Work out the finished part from the listing and answer in its coordinate system (mm). A direction names the side the tool comes from. Give positions to 0.01 mm unless a question says otherwise; leave off trailing zeros. Loops run counter-clockwise (first coordinate to the right, second up) from the corner with the lowest first, then second, coordinate; pieces in that order, holes last. Notation, with made-up numbers: M 88,-19.5 L 105,-19.5 A28 ccw 105,-0.5 Z; hole C 14,-39 d1. An arc over 180 degrees is marked long. Answer as a JSON object with one key per item and string values. Group by question number.
```python
from build123d import *

# Parameters (mm, degrees)
BOSS_EXTRUDE1_DEPTH = 3
BOSS_EXTRUDE2_DEPTH = 41
BOSS_EXTRUDE3_DEPTH = 2
SKETCH5_R           = 4.5
CUT_EXTRUDE1_DEPTH  = 2


with BuildPart() as part:
    # Sketch1 → Boss-Extrude1 (new body)
    with BuildSketch(Plane(origin=(0, 0, 0), x_dir=(1, 0, 0), z_dir=(0, 1, 0))):
        with BuildLine():
            Line((1.5, 0), (28.5, 0))
            ThreePointArc((28.5, 0), (29.560660172, 0.439339828), (30, 1.5))
            Line((30, 1.5), (30, 18.5))
            ThreePointArc((30, 18.5), (29.560660172, 19.560660172), (28.5, 20))
            Line((28.5, 20), (1.5, 20))
            ThreePointArc((1.5, 20), (0.439339828, 19.560660172), (0, 18.5))
            Line((0, 18.5), (0, 1.5))
            ThreePointArc((0, 1.5), (0.439339828, 0.439339828), (1.5, 0))
        make_face()
    extrude(amount=BOSS_EXTRUDE1_DEPTH)

    # Sketch3 → Boss-Extrude2 (add)
    with BuildSketch(Plane(origin=(0, 3, 0), x_dir=(1, 0, 0), z_dir=(0, 1, 0))):
        with BuildLine():
            Line((10.5, 5), (19.5, 5))
            ThreePointArc((19.5, 5), (19.853553391, 5.146446609), (20, 5.5))
            Line((20, 5.5), (20, 14.5))
            ThreePointArc((20, 14.5), (19.853553391, 14.853553391), (19.5, 15))
            Line((19.5, 15), (10.5, 15))
            ThreePointArc((10.5, 15), (10.146446609, 14.853553391), (10, 14.5))
            Line((10, 14.5), (10, 5.5))
            ThreePointArc((10, 5.5), (10.146446609, 5.146446609), (10.5, 5))
        make_face()
    extrude(amount=BOSS_EXTRUDE2_DEPTH)

    # Sketch4 → Boss-Extrude3 (add)
    with BuildSketch(Plane(origin=(0, 44, 0), x_dir=(1, 0, 0), z_dir=(0, 1, 0))):
        with BuildLine():
            Line((33, -22.5), (-3, -22.5))
            ThreePointArc((-3, -22.5), (-4.414213562, -21.914213562), (-5, -20.5))
            Line((-5, -20.5), (-5, 40.5))
            ThreePointArc((-5, 40.5), (-4.414213562, 41.914213562), (-3, 42.5))
            Line((-3, 42.5), (33, 42.5))
            ThreePointArc((33, 42.5), (34.414213562, 41.914213562), (35, 40.5))
            Line((35, 40.5), (35, -20.5))
            ThreePointArc((35, -20.5), (34.414213562, -21.914213562), (33, -22.5))
        make_face()
    extrude(amount=BOSS_EXTRUDE3_DEPTH)

    # Sketch5 → Cut-Extrude1 (cut)
    with BuildSketch(Plane(origin=(0, 46, 0), x_dir=(1, 0, 0), z_dir=(0, 1, 0))):
        with Locations(Location((15, 27.5, 0), (0, 0, 270))):
            Circle(SKETCH5_R)
        with Locations(Location((15, -7.5, 0), (0, 0, 270))):
            Circle(SKETCH5_R)
    extrude(amount=-CUT_EXTRUDE1_DEPTH, mode=Mode.SUBTRACT)


solid = part.part
```
Item 1: A cutting plane is placed at C-C (x = 15). Determine the outline of the cut face in (y, z), and give its area (3 significant figures).
Item 2: For a pull along Y with two mould halves and no side action, classify faces 4 (the cylindrical face through (34.43, 44.99, 21.9)), 5 (the flat face through (15, 0, -10)), 6 (the flat face through (15, 23, -15)) as pulls with the +Y half, pulls with the -Y half, needs draft (parallel to the pull), parting line crosses it, or undercut.
Item 3: A cutting plane is placed at A-A (x = 22.5). Determine the outline of the cut face in (y, z).
Item 4: A cutting plane is placed at B-B (z = -27.5). Determine the outline of the cut face in (x, y).
Item 5: Given pin 1 Ø12 at (y, z) = (12.5, -21.5) entering from +X; pin 2 Ø1.5 at (y, z) = (1, -10) entering from +X; pin 3 Ø2.5 at (y, z) = (29, -9) entering from -X; pin 4 Ø10 at (x, y) = (18, 34) entering from +Z, each flat-ended and moving along its own axis, determine where each tip first touches the part or whether it passes through.
Item 6: A tool of negligible diameter and unlimited length cuts with its end or side. For faces 1 (the cylindrical face through (29.55, 1.48, -0.43)), 2 (the cylindrical face through (0.43, 1.48, -0.45)), 3 (the flat face through (0, 1, -10)), from which of +Z, -Z, +X, -X, +Y, -Y can it reach the whole face along a straight path? Write none if from no direction.
Item 7: A cutting plane is placed at D-D (y = 41). Determine the outline of the cut face in (x, z), and give its area (3 significant figures).
Item 8: Find the intervals of material crossed by probe 1 along X at (y, z) = (45.3, -27.5); probe 2 along Y at (x, z) = (1.5, -16); probe 3 along Y at (x, z) = (7, 0.5), in increasing order. Write a range as [from, to].
The answers:
{
 "1": {"outline": "M 0,-20 L 3,-20 L 3,-15 L 44,-15 L 44,-23 L 46,-23 L 46,3 L 44,3 L 44,-5 L 3,-5 L 3,0 L 0,0 Z; M 44,-42.5 L 46,-42.5 L 46,-32 L 44,-32 Z; M 44,12 L 46,12 L 46,22.5 L 44,22.5 Z", "area": "564 mm^2"},
 "2": {"face 4": "needs draft", "face 5": "pulls with the -Y half", "face 6": "undercut"},
 "3": {"outline": "M 0,-20 L 3,-20 L 3,0 L 0,0 Z; M 44,-42.5 L 46,-42.5 L 46,22.5 L 44,22.5 Z"},
 "4": {"outline": "M -5,44 L 10.5,44 L 10.5,46 L -5,46 Z; M 19.5,44 L 35,44 L 35,46 L 19.5,46 Z"},
 "5": {"pin 1": "passes through", "pin 2": "stops at x = 30", "pin 3": "stops at x = 10", "pin 4": "stops at z = -5"},
 "6": {"face 1": "+Z, +X, -Y", "face 2": "+Z, -X, -Y", "face 3": "+Z, -Z, -X, -Y"},
 "7": {"outline": "M 10,-14.5 A0.5 ccw 10.5,-15 L 19.5,-15 A0.5 ccw 20,-14.5 L 20,-5.5 A0.5 ccw 19.5,-5 L 10.5,-5 A0.5 ccw 10,-5.5 Z", "area": "99.8 mm^2"},
 "8": {"probe 1": "x = [-5, 10.5], [19.5, 35]", "probe 2": "y = [0, 3], [44, 46]", "probe 3": "y = [44, 46]"}
}
